```python
from build123d import *

# Parameters (mm, degrees)
EXTRUDE_9_DEPTH      = 40
EXTRUDE_START        = 3
EXTRUDE_10_DEPTH     = 3
SKETCH_11_R          = 10
CUT_EXTRUDE_1_DEPTH  = 3
EXTRUDE_11_DEPTH     = 10
SKETCH_21_W          = 13.008941923
SKETCH_21_H          = 10
CUT_EXTRUDE_9_DEPTH  = 65.045413014
EXTRUDE_12_REACH     = 65.691
SKETCH_23_W          = 10
SKETCH_23_H          = 3
FILLET_1_R           = 3
FILLET_2_R           = 3
FILLET_3_DEPTH       = 10
CUT_EXTRUDE_10_REACH = 63.068


with BuildPart() as part:
    # 草图5 → 凸台-拉伸9 (new body)
    with BuildSketch(Plane.XY):
        with BuildLine():
            Line((0, 16.799900253), (-39.976031579, 16.799900253))
            Line((-39.976031579, 16.799900253), (-39.976031579, 12.499900253))
            Line((-39.976031579, 12.499900253), (-29.976031579, 12.499900253))
            Line((-29.976031579, 12.499900253), (0.295610531, 14.79704749))
            ThreePointArc((0.295610531, 14.79704749), (14.79704749, -0.295610531), (-0.295610531, -14.79704749))
            Line((-0.295610531, -14.79704749), (-29.976031579, -12.499900253))
            Line((-29.976031579, -12.499900253), (-39.976031579, -12.499900253))
            Line((-39.976031579, -12.499900253), (-39.976031579, -16.799900253))
            Line((-39.976031579, -16.799900253), (0, -16.799900253))
            ThreePointArc((0, -16.799900253), (16.799900253, 0), (0, 16.799900253))
        make_face()
    extrude(amount=EXTRUDE_9_DEPTH)

    # 草图10 → 凸台-拉伸10 (add)
    with BuildSketch(Plane(origin=(0, 0, 0), x_dir=(-1, 0, 0), z_dir=(0, 0, -1)).offset(EXTRUDE_START)):
        with BuildLine():
            Line((0, -16.799900253), (39.976031579, -16.799900253))
            Line((39.976031579, -16.799900253), (39.976031579, 16.799900253))
            Line((39.976031579, 16.799900253), (0, 16.799900253))
            ThreePointArc((0, 16.799900253), (-16.799900253, 0), (0, -16.799900253))
        make_face()
    extrude(amount=-EXTRUDE_10_DEPTH)

    # 草图11 → 切除-拉伸1 (cut)
    with BuildSketch(Plane(origin=(0, 0, -3), x_dir=(-1, 0, 0), z_dir=(0, 0, -1))):
        Circle(SKETCH_11_R)
    extrude(amount=-CUT_EXTRUDE_1_DEPTH, mode=Mode.SUBTRACT)

    # 草图18 → 凸台-拉伸11 (add)
    with BuildSketch(Plane.XY):
        with BuildLine():
            Line((-39.976031579, -12.499900253), (-29.976031579, -12.499900253))
            Line((-29.976031579, -12.499900253), (-20.032968003, -13.26945406))
            Line((-20.032968003, -13.26945406), (-0.295610531, -14.79704749))
            ThreePointArc((-0.295610531, -14.79704749), (14.79704749, -0.295610531), (0.295610531, 14.79704749))
            Line((0.295610531, 14.79704749), (-17.004384343, 13.484246708))
            Line((-17.004384343, 13.484246708), (-17.004384343, 5))
            Line((-17.004384343, 5), (-8.660254038, 5))
            ThreePointArc((-8.660254038, 5), (10, 0), (-8.660254038, -5))
            Line((-8.660254038, -5), (-20, -5))
            Line((-20, -5), (-29.976031579, -5))
            Line((-29.976031579, -5), (-29.976031579, 5))
            Line((-29.976031579, 5), (-29.976031579, 12.499900253))
            Line((-29.976031579, 12.499900253), (-39.976031579, 12.499900253))
            Line((-39.976031579, 12.499900253), (-39.976031579, -12.499900253))
        make_face()
    extrude(amount=EXTRUDE_11_DEPTH)

    # 草图21 → 切除-拉伸9 (cut, through all)
    with BuildSketch(Plane(origin=(-1.114744508, 14.690023458, 0), x_dir=(0.9971331498487674, 0.07566691134621262, 0), z_dir=(0.07566691134621262, -0.9971331498487674, 0))):
        with Locations((-22.439794983, 5)):
            Rectangle(SKETCH_21_W, SKETCH_21_H)
    extrude(amount=-CUT_EXTRUDE_9_DEPTH, mode=Mode.SUBTRACT)

    # 草图23 → 凸台-拉伸12 (add, up to next)
    with BuildSketch(Plane.XZ.offset(-12.499900253), mode=Mode.PRIVATE) as extrude_12_sk1:
        with Locations((-34.976031579, 38.5)):
            Rectangle(SKETCH_23_W, SKETCH_23_H)
    extrude_12_tool1 = extrude(extrude_12_sk1.sketch, amount=EXTRUDE_12_REACH, mode=Mode.PRIVATE) - part.part
    add(extrude_12_tool1.solids().sort_by_distance((-34.976032, 12.4999, 38.5))[0])

    # 圆角1
    # the kernel refuses this fillet: 3 mm, written as the material it takes off along each edge
    with BuildSketch(Plane(origin=(-47.476031579, -16.799900253, 40), x_dir=(0, 0, -1), z_dir=(1, 0, 0)), Plane(origin=(0, 16.799900253, 40), x_dir=(0, 0, -1), z_dir=(-1, 0, 0))) as fillet_1_piece_1:
        with BuildLine():
            CenterArc((FILLET_1_R, FILLET_1_R), FILLET_1_R, 180, 90)
            Line((0, FILLET_1_R), (0, 0))
            Line((0, 0), (FILLET_1_R, 0))
        make_face()
    extrude(amount=47.476031579, mode=Mode.SUBTRACT)
    with BuildSketch(Plane(origin=(0, 0, 40), x_dir=(0, -1, 0), z_dir=(-1, 0, 0))) as fillet_1_piece_2:
        with BuildLine():
            CenterArc((16.799900253 - FILLET_1_R, -FILLET_1_R), FILLET_1_R, 0, 90)
            Line((16.799900253, -FILLET_1_R), (16.799900253, 0))
            Line((16.799900253, 0), (16.799900253 - FILLET_1_R, 0))
        make_face()
    revolve(axis=Axis((0, 0, 40), (0, 0, 1)), revolution_arc=180, mode=Mode.SUBTRACT)

    # 圆角2
    fillet_2_edges = [part.edges().sort_by_distance(p)[0] for p in [
        (-39.976031579, 0, 40),
        (-39.976031579, -16.799900253, 17),
        (-39.976031579, 16.799900253, 17),
        (-39.976031579, 15.921220597, 39.121320344),
        (-39.976031579, -15.921220597, 39.121320344),
        (16.799900253, 0, -3),
        (-19.988015789, -16.799900253, -3),
        (-39.976031579, 0, -3),
        (-19.988015789, 16.799900253, -3),
    ]]
    fillet(fillet_2_edges, radius=FILLET_2_R - 0.0001)  # a hair under: the kernel refuses the full size

    # 圆角3: read off the stored shape, not the designer's step
    # 圆角3 outline → 圆角3 (cut)
    with BuildSketch(Plane.XY):
        with BuildLine():
            Line((-17.004384343, 5), (-8.660254038, 5))
            ThreePointArc((-8.660254038, 5), (-14.43892528, 8.102315607), (-17.052465962, 14.117862844))
            Line((-17.052465962, 14.117862844), (-17.004384343, 13.484246708))
            Line((-17.004384343, 13.484246708), (-17.004384343, 5))
        make_face()
    extrude(amount=FILLET_3_DEPTH, mode=Mode.SUBTRACT)

    # 草图27 → 切除-拉伸10 (cut, up to next)
    with BuildSketch(Plane(origin=(0, 0, -3), x_dir=(-1, 0, 0), z_dir=(0, 0, -1)), mode=Mode.PRIVATE) as cut_extrude_10_sk1:
        with BuildLine():
            ThreePointArc((9.928, -1.197838052), (10, 0), (9.928, 1.197838052))
            ThreePointArc((9.928, 1.197838052), (11.2, 0), (9.928, -1.197838052))
        make_face()
    cut_extrude_10_tool1 = extrude(cut_extrude_10_sk1.sketch, amount=-CUT_EXTRUDE_10_REACH, mode=Mode.PRIVATE) & part.part
    # 草图27 → 切除-拉伸10 (cut, up to next)
    with BuildSketch(Plane(origin=(0, 0, -3), x_dir=(-1, 0, 0), z_dir=(0, 0, -1)), mode=Mode.PRIVATE) as cut_extrude_10_sk2:
        with BuildLine():
            ThreePointArc((-6.173156714, -7.867155533), (-7.919595949, -7.919595949), (-7.867155533, -6.173156714))
            ThreePointArc((-7.867155533, -6.173156714), (-7.071067812, -7.071067812), (-6.173156714, -7.867155533))
        make_face()
    cut_extrude_10_tool2 = extrude(cut_extrude_10_sk2.sketch, amount=-CUT_EXTRUDE_10_REACH, mode=Mode.PRIVATE) & part.part
    # 草图27 → 切除-拉伸10 (cut, up to next)
    with BuildSketch(Plane(origin=(0, 0, -3), x_dir=(-1, 0, 0), z_dir=(0, 0, -1)), mode=Mode.PRIVATE) as cut_extrude_10_sk3:
        with BuildLine():
            ThreePointArc((-7.867155533, 6.173156714), (-7.071067812, 7.071067812), (-6.173156714, 7.867155533))
            ThreePointArc((-6.173156714, 7.867155533), (-7.919595949, 7.919595949), (-7.867155533, 6.173156714))
        make_face()
    cut_extrude_10_tool3 = extrude(cut_extrude_10_sk3.sketch, amount=-CUT_EXTRUDE_10_REACH, mode=Mode.PRIVATE) & part.part
    add(cut_extrude_10_tool1.solids().sort_by_distance((-10.496108, 0, -3))[0], mode=Mode.SUBTRACT)
    add(cut_extrude_10_tool2.solids().sort_by_distance((7.421869, -7.421869, -3))[0], mode=Mode.SUBTRACT)
    add(cut_extrude_10_tool3.solids().sort_by_distance((7.421869, 7.421869, -3))[0], mode=Mode.SUBTRACT)


solid = part.part
```
The model under review builds one solid part; all positions refer to its coordinate system, in mm. A direction names the side the tool comes from. Round coordinates to 2 decimals unless told otherwise and drop trailing zeros. Write each loop counter-clockwise with the first axis right and the second up, starting at its lowest first coordinate (ties: lowest second). Pieces come first, ordered by that corner, then holes. Notation, with made-up numbers: M 28.5,77.25 L 45.5,77.25 A24 cw 45.5,102.25 Z; hole C 21,-40 d7. An arc over 180 degrees is marked long. Use CSV: the item, a comma, the result in double quotes. Start each with the question number.
(1) Clearance check with flat-ended pins moving along their axes: P1, Ø3, axis at x = -20, z = 6, coming from the +Y side; P2, Ø5, axis at x = 4.5, z = 30, coming from the +Y side; P3, Ø1.3, axis at x = -25, y = 15, coming from the -Z side. State where each tip first meets the part, or that it passes through.
(2) Tool access review of faces 5 (the face through (-18, -16.8, 18)), 6 (the face through (14.8, 0, 24.7)), 7 (the face through (-13, -6, 10)): name each direction out of +Z, -Z, +X, -X, +Y, -Y from which nothing blocks a thin tool from reaching the whole face with its end or side.
(3) For line 1 along Y through (x, z) = (-32, 28); line 2 along Z through (x, y) = (-29, 5); line 3 along Z through (x, y) = (-4, 10.5), list the stretches that pass through material, from the lowest coordinate up.
(4) We need section C-C, the plane y = 0. State how many separate pieces and enclosed holes the cut face has, then the cut area to 3 significant figures.
(5) We need section B-B, the plane z = 25. State the section outline as (x, y) points.
(6) The part is to be moulded in two halves that separate along Y. For faces 1 (the face through (-15.052, 13.632, 24.79)), 2 (the face through (-39.12, 0.19, -2.1)), 3 (the face through (-35, 0, 37)), 4 (the face through (-18.75, -15.9, 39.14)), say which applies: +Y half, -Y half, draft (parallel to the pull), parting line (faces both ways), or undercut.
(7) We need section D-D, the plane x = -12. State the section outline as (y, z) points, then the cut area to 3 significant figures.
Findings:
1,P1,"y = -5"
1,P2,"y = 16.68"
1,P3,"z = -2.95"
2,face 5,"+Z, -Z, +X, -X, -Y"
2,face 6,"+Z"
2,face 7,"none"
3,line 1,"-16.8 to -12.5, 12.5 to 16.8"
3,line 2,"-3 to 0"
3,line 3,"-3 to 10"
4,separate pieces,"3"
4,enclosed holes,"0"
4,area,"357 mm^2"
5,outline,"M -39.98,-13.8 A3 ccw -36.98,-16.8 L 0,-16.8 A16.8 ccw 0,16.8 L -36.98,16.8 A3 ccw -39.98,13.8 L -39.98,12.5 L -29.98,12.5 L 0.3,14.8 A14.8 cw -0.3,-14.8 L -29.98,-12.5 L -39.98,-12.5 Z"
6,face 1,"undercut"
6,face 2,"draft"
6,face 3,"undercut"
6,face 4,"-Y half"
7,outline,"M -16.8,0 A3 ccw -13.8,-3 L 13.8,-3 A3 ccw 16.8,0 L 16.8,37 A3 ccw 13.86,40 L 13.86,10 L 6.17,10 L 6.17,0 L -5,0 L -5,10 L -13.89,10 L -13.89,40 A3 ccw -16.8,37 Z"
7,area,"493 mm^2"
